The listing builds one solid part. Answer for the finished solid, in the listing's coordinates (mm). A direction names the side the tool comes from. Coordinates: 2 decimals unless noted, no trailing zeros. Loops run counter-clockwise (first coordinate to the right, second up) from the corner with the lowest first, then second, coordinate; pieces in that order, holes last. Notation, with made-up numbers: M -7,34.25 L 50,34.25 A16 ccw 50,45.25 Z; hole C 6,55.25 d4. An arc over 180 degrees is marked long. Answer as a JSON object with one key per item and string values. Group by question number.
1. Given pin 1 (2 mm diameter, centred on x = 29.37, y = 48.54, fed in from +Z); pin 2 (5 mm diameter, centred on y = 7.5, z = -47, fed in from +X); pin 3 (1.5 mm diameter, centred on y = 1, z = -46, fed in from +X); pin 4 (4 mm diameter, centred on x = 13.5, y = 42.5, fed in from -Z), each flat-ended and moving along its own axis, determine where each tip first touches the part or whether it passes through.
2. A cutting plane is placed at C-C on y = -5.5. Give the vertices of the cut face in (x, z).
3. A cutting plane is placed at B-B on z = -63. Give the vertices of the cut face in (x, y), and give its area (3 significant figures).
4. Straight lines are drawn through the part: L1, parallel to X at y = 6.5, z = -13.5; L2, parallel to Y at x = -6.5, z = -62.5; L3, parallel to Z at x = 13.5, y = 25. For each, find the intervals that lie inside material, in ascending order.
5. For faces 1 (the face through (-6.35, -28, -3)), 2 (the face through (0, -19.404, -10)), 3 (the face through (45.138, -50.388, -36.386)), determine the directions among +Z, -Z, +X, -X, +Y, -Y from which every point of the face is accessible in a straight line to the end or side of a thin tool.
6. Determine the mould class of faces 4 (the face through (9, -1, -15.24)), 5 (the face through (7, -1, -12.7)), 6 (the face through (-57.488, 3.021, -33.81)) for opening direction Z: released by +Z, released by -Z, zero draft, split by the parting line, or undercut.
7. A cutting plane is placed at A-A on x = -4. Give the vertices of the cut face in (y, z).
8. A cutting plane is placed at D-D on x = 14.5. Give the vertices of the cut face in (y, z), and give its area (3 significant figures).
from build123d import *

# Parameters (mm, degrees)
SKETCH1_W           = 12.7
SKETCH1_H           = 6.35
BOSS_EXTRUDE1_DEPTH = 5.08
BOSS_EXTRUDE2_DEPTH = 63.5
BOSS_EXTRUDE3_DEPTH = 10.16
CUT_EXTRUDE1_DEPTH  = 7.62
SKETCH9_R           = 1.27
CUT_EXTRUDE2_DEPTH  = 5.08


with BuildPart() as part:
    # Sketch1 → Boss-Extrude1 (new body)
    with BuildSketch(Plane.XY):
        with BuildLine():
            Line((63.5, 56.7961272), (-63.5, 56.7961272))
            Line((-63.5, 56.7961272), (-51.304854459, -52.280570501))
            ThreePointArc((-51.304854459, -52.280570501), (-49.642976536, -55.502534499), (-46.25630987, -56.796126057))
            Line((-46.25630987, -56.796126057), (46.25630987, -56.796126057))
            ThreePointArc((46.25630987, -56.796126057), (49.642976536, -55.502534499), (51.304854459, -52.280570501))
            Line((51.304854459, -52.280570501), (63.5, 56.7961272))
        make_face()
        with Locations((0, -28.221126057)):
            Rectangle(SKETCH1_W, SKETCH1_H, mode=Mode.SUBTRACT)
    extrude(amount=-BOSS_EXTRUDE1_DEPTH)

    # Sketch2 → Boss-Extrude2 (add)
    with BuildSketch(Plane.XY.offset(-5.08)):
        with BuildLine():
            Line((51.304854459, -52.280570501), (63.5, 56.7961272))
            Line((63.5, 56.7961272), (58.388348603, 56.7961272))
            Line((58.388348603, 56.7961272), (46.761164329, -47.200570501))
            ThreePointArc((46.761164329, -47.200570501), (45.099286406, -50.422534499), (41.712619739, -51.716126057))
            Line((41.712619739, -51.716126057), (-41.712619739, -51.716126057))
            ThreePointArc((-41.712619739, -51.716126057), (-45.099286406, -50.422534499), (-46.761164329, -47.200570501))
            Line((-46.761164329, -47.200570501), (-58.388348603, 56.7961272))
            Line((-58.388348603, 56.7961272), (-63.5, 56.7961272))
            Line((-63.5, 56.7961272), (-51.304854459, -52.280570501))
            ThreePointArc((-51.304854459, -52.280570501), (-49.642976536, -55.502534499), (-46.25630987, -56.796126057))
            Line((-46.25630987, -56.796126057), (46.25630987, -56.796126057))
            ThreePointArc((46.25630987, -56.796126057), (49.642976536, -55.502534499), (51.304854459, -52.280570501))
        make_face()
    extrude(amount=-BOSS_EXTRUDE2_DEPTH)

    # Sketch4 → Boss-Extrude3 (add)
    with BuildSketch(Plane(origin=(0, 0, -5.08), x_dir=(-1, 0, 0), z_dir=(0, 0, -1))):
        Polygon((-20.319997003, 44.0961272), (-20.319997003, -19.4038728), (20.320002997, -19.4038728), align=None)
    extrude(amount=BOSS_EXTRUDE3_DEPTH)

    # Sketch7 → Cut-Extrude1 (cut)
    with BuildSketch(Plane(origin=(0, 0, -12.7), x_dir=(-1, 0, 0), z_dir=(0, 0, -1))):
        Polygon((18.694402997, -16.8638728), (-17.779997003, -16.8638728), (-17.779997003, 40.1273772), align=None)
    extrude(amount=-CUT_EXTRUDE1_DEPTH, mode=Mode.SUBTRACT)

    # Sketch9 → Cut-Extrude2 (cut)
    with BuildSketch(Plane.XY):
        with Locations((29.36937484, 48.5411272)):
            Circle(SKETCH9_R)
        with Locations((-29.36937484, 48.5411272)):
            Circle(SKETCH9_R)
        with Locations((29.36937484, -23.848871657)):
            Circle(SKETCH9_R)
        with Locations((-29.36937484, -23.848871657)):
            Circle(SKETCH9_R)
    extrude(amount=-CUT_EXTRUDE2_DEPTH, mode=Mode.SUBTRACT)


solid = part.part
From the geometry:
{
 "1": {"pin 1": "passes through", "pin 2": "stops at x = 58.27", "pin 3": "stops at x = 57.35", "pin 4": "stops at z = -5.08"},
 "2": {"outline": "M -56.54,-68.58 L -51.42,-68.58 L -51.42,-5.08 L 17.78,-5.08 L 17.78,-12.7 L -11.42,-12.7 L -11.42,-15.24 L 20.32,-15.24 L 20.32,-5.08 L 51.42,-5.08 L 51.42,-68.58 L 56.54,-68.58 L 56.54,0 L -56.54,0 Z"},
 "3": {"outline": "M -63.5,56.8 L -51.3,-52.28 A5.08 ccw -46.26,-56.8 L 46.26,-56.8 A5.08 ccw 51.3,-52.28 L 63.5,56.8 L 58.39,56.8 L 46.76,-47.2 A5.08 cw 41.71,-51.72 L -41.71,-51.72 A5.08 cw -46.76,-47.2 L -58.39,56.8 Z", "area": "1,630 mm²"},
 "4": {"L1": "x = -57.88 to -52.77, -3.74 to 20.32, 52.77 to 57.88", "L2": "y = -56.8 to -51.72", "L3": "z = -15.24 to -12.7, -5.08 to 0"},
 "5": {"face 1": "+Z, -Z", "face 2": "-Z", "face 3": "-Z, +Y"},
 "6": {"face 4": "released by -Z", "face 5": "undercut", "face 6": "zero draft"},
 "7": {"outline": "M -56.8,-68.58 L -51.72,-68.58 L -51.72,-5.08 L -31.4,-5.08 L -31.4,0 L -56.8,0 Z; M -25.05,-5.08 L -19.4,-5.08 L -19.4,-15.24 L 6.1,-15.24 L 6.1,-12.7 L -16.86,-12.7 L -16.86,-5.08 L 56.8,-5.08 L 56.8,0 L -25.05,0 Z"},
 "8": {"outline": "M -56.8,-68.58 L -51.72,-68.58 L -51.72,-5.08 L -19.4,-5.08 L -19.4,-15.24 L 35,-15.24 L 35,-12.7 L -16.86,-12.7 L -16.86,-5.08 L 56.8,-5.08 L 56.8,0 L -56.8,0 Z", "area": "1,060 mm²"}
}
